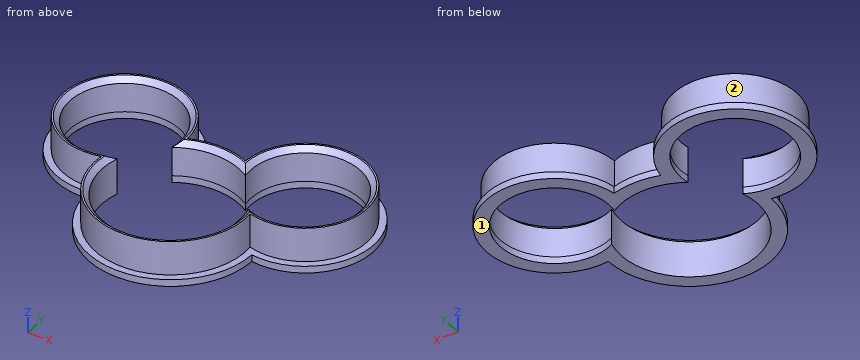
```python
from build123d import *

# Parameters (mm, degrees)
PAD_DEPTH       = 10
SKETCH001_R     = 20
POCKET_DEPTH    = 10
SKETCH002_R     = 16
POCKET001_DEPTH = 10
CHAMFER_SIZE    = 1.5
CHAMFER001_SIZE = 1.5
CHAMFER002_SIZE = 1.5
CHAMFER003_SIZE = 1.5
PAD001_DEPTH    = 2


with BuildPart() as part:
    # Sketch → Pad (new body)
    with BuildSketch(Plane.XY):
        with BuildLine():
            ThreePointArc((38.5386550517, 16.614400785), (57.6494681052, 44.7125163297), (25.1916455851, 34.6518488576))
            ThreePointArc((25.1916455851, 34.6518488576), (16.6527682137, 36.3765542054), (8.1138908423, 34.6518488576))
            ThreePointArc((8.1138908423, 34.6518488576), (-24.3439316777, 44.7125163297), (-5.2331186243, 16.614400785))
            ThreePointArc((-5.2331186243, 16.614400785), (16.6527682137, -7.6234457946), (38.5386550517, 16.614400785))
        make_face()
    extrude(amount=PAD_DEPTH)

    # Sketch001 (on Face6 of Pad) → Pocket (cut)
    with BuildSketch(Plane.XY.offset(10)):
        with Locations((16.6527682137, 14.3765542054)):
            Circle(SKETCH001_R)
    extrude(amount=-POCKET_DEPTH, mode=Mode.SUBTRACT)

    # Sketch002 (on Face5 of Pocket) → Pocket001 (cut)
    with BuildSketch(Plane.XY.offset(10)):
        with Locations((-9.8745081866, 34.0057061682)):
            Circle(SKETCH002_R)
        with Locations((43.1800446141, 34.0057061682)):
            Circle(SKETCH002_R)
    extrude(amount=-POCKET001_DEPTH, mode=Mode.SUBTRACT)

    # Chamfer
    chamfer_edges = [part.edges().sort_by_distance(p)[0] for p in [
        (41.78641, 49.944896, 10),
    ]]
    chamfer(chamfer_edges, length=CHAMFER_SIZE)

    # Chamfer001
    chamfer001_edges = [part.edges().sort_by_distance(p)[0] for p in [
        (36.574516, 16.144027, 10),
    ]]
    chamfer(chamfer001_edges, length=CHAMFER001_SIZE)

    # Chamfer002
    chamfer002_edges = [part.edges().sort_by_distance(p)[0] for p in [
        (15.703375, 34.354008, 10),
    ]]
    chamfer(chamfer002_edges, length=CHAMFER002_SIZE)

    # Chamfer003
    chamfer003_edges = [part.edges().sort_by_distance(p)[0] for p in [
        (-22.998023, 43.158485, 10),
    ]]
    chamfer(chamfer003_edges, length=CHAMFER003_SIZE)

    # Sketch004 (on Face20 of Chamfer003) → Pad001 (join)
    with BuildSketch(Plane(origin=(0, 0, 0), x_dir=(1, 0, 0), z_dir=(0, 0, -1))):
        with BuildLine():
            ThreePointArc((40.6518458567, -14.1661444028), (16.6527682137, 9.6234457946), (-7.3463094293, -14.1661444028))
            ThreePointArc((-7.3463094293, -14.1661444028), (-25.951645399, -45.9021619032), (9.8373328664, -37.3885041668))
            ThreePointArc((9.8373328664, -37.3885041668), (16.6527682137, -38.3765542054), (23.4682035611, -37.3885041668))
            ThreePointArc((23.4682035611, -37.3885041668), (59.2571818264, -45.9021619032), (40.6518458567, -14.1661444028))
        make_face()
        with BuildLine():
            ThreePointArc((35.917730039, -19.7488205682), (16.6527682137, 5.6234457946), (-2.6121936115, -19.7488205682))
            ThreePointArc((-2.6121936115, -19.7488205682), (-22.7362179565, -43.5228707562), (5.8827146104, -31.2290301476))
            ThreePointArc((5.8827146104, -31.2290301476), (16.6527682137, -34.3765542054), (27.422821817, -31.2290301476))
            ThreePointArc((27.422821817, -31.2290301476), (56.041754384, -43.5228707562), (35.917730039, -19.7488205682))
        make_face(mode=Mode.SUBTRACT)
    extrude(amount=PAD001_DEPTH)


solid = part.part
```
The listing builds one solid part. Answer for the finished solid, in the listing's coordinates (mm). Face numbers are marked on the shaded views. Coordinates: 2 decimals unless noted, no trailing zeros. Write each loop counter-clockwise with the first axis right and the second up, starting at its lowest first coordinate (ties: lowest second). Pieces come first, ordered by that corner, then holes. Notation, with made-up numbers: M -5,10.5 L 54,10.5 A21 cw 54,27.5 Z; hole C 35,6.5 d7. An arc over 180 degrees is marked long. Use a Markdown table: item, result. Add a question column.
1. Section A-A (z = 1) is taken. Give the vertices of the cut face in (x, y), plus the area to 3 significant figures.
2. For a pull along X with two mould halves and no side action, classify the marked faces 1 and 2 as +X half, -X half, draft (parallel to the pull), parting line (faces both ways), or undercut.
3. Given P1, Ø1.5, axis at y = 7.5, z = 8, coming from the -X side; P2, Ø4, axis at y = 7.5, z = 0, coming from the -X side; P3, Ø2, axis at y = -0.5, z = 7, coming from the +X side, each flat-ended and moving along its own axis, determine where each tip first touches the part or whether it passes through.
4. Straight lines are drawn through the part: line 1 along X through (y, z) = (44, 6.5); line 2 along X through (y, z) = (45, 8.25); line 3 along X through (y, z) = (30, 1.5). For each, find the intervals that lie inside material, in ascending order. Write a range as [from, to].
5. Section B-B (y = 40) is taken. Count the separate pieces of the cut face and the enclosed holes in it, plus the area to 3 significant figures.
Data:
| question | item | result |
|---|---|---|
| 1 | outline | M -5.23,16.61 A22 ccw long 38.54,16.61 A18 ccw long 25.19,34.65 A22 ccw 8.11,34.65 A18 ccw long Z; hole M -2.61,19.75 A20 ccw long 35.92,19.75 A16 ccw long 27.42,31.23 A20 ccw 5.88,31.23 A16 ccw long Z |
| 1 | area | 535 mm2 |
| 2 | face 1 | draft |
| 2 | face 2 | undercut |
| 3 | P1 | stops at x = -4.48 |
| 3 | P2 | stops at x = -6.85 |
| 3 | P3 | stops at x = 33.72 |
| 4 | line 1 | x = [-24.84, -22.37], [2.62, 5.1], [28.21, 30.69], [55.67, 58.15] |
| 4 | line 2 | x = [-24.13, -21.5], [1.75, 4.38], [28.93, 31.56], [54.8, 57.43] |
| 4 | line 3 | x = [-27.42, -25.36], [58.67, 60.73] |
| 5 | separate pieces | 4 |
| 5 | enclosed holes | 0 |
| 5 | area | 115 mm2 |
